Read the model definition and answer for the solid it produces. Units are mm, in the model's axes. A direction names the side the tool comes from. Give positions to 0.01 mm unless a question says otherwise; leave off trailing zeros. Write each loop counter-clockwise with the first axis right and the second up, starting at its lowest first coordinate (ties: lowest second). Pieces come first, ordered by that corner, then holes. Notation, with made-up numbers: M 15,70 L 58,70 A18 cw 58,89 Z; hole C 10,-34.5 d5. An arc over 180 degrees is marked long. Put each result on its own line as item: value.
from build123d import *

# Parameters (mm, degrees)
SKETCH1_R           = 16.66875
BOSS_EXTRUDE1_DEPTH = 3.175
SKETCH2_R           = 16.66875
SKETCH2_R_2         = 13.49375
BOSS_EXTRUDE2_DEPTH = 53.975
SKETCH7_R           = 6.985
CUT_EXTRUDE1_DEPTH  = 62.82084562
SKETCH12_R          = 14.2875
BOSS_EXTRUDE7_DEPTH = 25.4
CUT_EXTRUDE2_REACH  = 63.821
SKETCH9_W           = 12.7
SKETCH9_H           = 11.43
SKETCH9_W_2         = 6.35
SKETCH9_H_2         = 1.6002
SKETCH9_W_3         = 152.4
SKETCH9_H_3         = 3.175
CIRPATTERN2_COUNT   = 4
SKETCH5_R           = 2.5527
SKETCH6_R           = 5.715
CIRPATTERN1_COUNT   = 4


with BuildPart() as part:
    # Sketch1 → Boss-Extrude1 (new body)
    with BuildSketch(Plane(origin=(0, 0, 0), x_dir=(1, 0, 0), z_dir=(0, 1, 0))):
        with Locations(Location((0, 0, 0), (0, 0, 270))):
            Circle(SKETCH1_R)
    extrude(amount=BOSS_EXTRUDE1_DEPTH)

    # Sketch2 → Boss-Extrude2 (add)
    with BuildSketch(Plane(origin=(0, 3.175, 0), x_dir=(1, 0, 0), z_dir=(0, 1, 0))):
        with Locations(Location((0, 0, 0), (0, 0, 270))):
            Circle(SKETCH2_R)
        with Locations(Location((0, 0, 0), (0, 0, 270))):
            Circle(SKETCH2_R_2, mode=Mode.SUBTRACT)
    extrude(amount=BOSS_EXTRUDE2_DEPTH)

    # Sketch7 → Cut-Extrude1 (cut, through all)
    with BuildSketch(Plane.XZ):
        with Locations(Location((0, 0, 0), (0, 0, 270))):
            Circle(SKETCH7_R)
    extrude(amount=-CUT_EXTRUDE1_DEPTH, mode=Mode.SUBTRACT)

    # Sketch12 → Boss-Extrude7 (add)
    with BuildSketch(Plane(origin=(0, 31.75, 0), x_dir=(1, 0, 0), z_dir=(0, 1, 0))):
        Circle(SKETCH12_R)
    extrude(amount=BOSS_EXTRUDE7_DEPTH)

    # Cut-Loft2: read off the stored shape, not the designer's step
    # Cut-Loft2: loft between two sections, ruled curve by curve
    cut_loft2_from = [
        Edge.make_bspline([(-0.505569823, 57.15, -10.307628823), (20.109687823, 57.15, -11.318768468), (21.120827469, 57.15, 9.296489178), (0.505569823, 57.15, 10.307628823), (-20.109687823, 57.15, 11.318768468), (-21.120827469, 57.15, -9.296489178), (-0.505569823, 57.15, -10.307628823)], [0, 0, 0, 0, 0.5, 0.5, 0.5, 1, 1, 1, 1], 3, [1, 0.333333333, 0.333333333, 1, 0.333333333, 0.333333333, 1]),
    ]
    cut_loft2_to = [
        Edge.make_bspline([(-3.365363271, 31.75, -5.384870477), (7.404377683, 31.75, -12.115597019), (14.135104225, 31.75, -1.345856065), (3.365363271, 31.75, 5.384870477), (-7.404377683, 31.75, 12.115597019), (-14.135104225, 31.75, 1.345856065), (-3.365363271, 31.75, -5.384870477)], [0, 0, 0, 0, 0.5, 0.5, 0.5, 1, 1, 1, 1], 3, [1, 0.333333333, 0.333333333, 1, 0.333333333, 0.333333333, 1]),
    ]
    cut_loft2 = Solid(Shell([*[Face.make_surface_from_curves(cut_loft2_from[k], cut_loft2_to[k]) for k in range(1)], Face(Wire(cut_loft2_from)), Face(Wire(cut_loft2_to))]))
    add(cut_loft2, mode=Mode.SUBTRACT)

    # Sketch9 → Cut-Extrude2 (cut, up to next)
    with BuildSketch(Plane(origin=(0, 0, 0), x_dir=(0, -1, 0), z_dir=(-0.7071067811865488, 0, 0.7071067811865464)), mode=Mode.PRIVATE) as cut_extrude2_sk1:
        with Locations((-9.52754, 0)):
            Rectangle(SKETCH9_W, SKETCH9_H)
    cut_extrude2_tool1 = extrude(cut_extrude2_sk1.sketch, amount=-CUT_EXTRUDE2_REACH, mode=Mode.PRIVATE) & part.part
    # Sketch9 → Cut-Extrude2 (cut, up to next)
    with BuildSketch(Plane(origin=(0, 0, 0), x_dir=(0, -1, 0), z_dir=(-0.7071067811865488, 0, 0.7071067811865464)), mode=Mode.PRIVATE) as cut_extrude2_sk2:
        with Locations((-22.225, 0)):
            Rectangle(SKETCH9_W_2, SKETCH9_H_2)
    cut_extrude2_tool2 = extrude(cut_extrude2_sk2.sketch, amount=-CUT_EXTRUDE2_REACH, mode=Mode.PRIVATE) & part.part
    # Sketch9 → Cut-Extrude2 (cut, up to next)
    with BuildSketch(Plane(origin=(0, 0, 0), x_dir=(0, -1, 0), z_dir=(-0.7071067811865488, 0, 0.7071067811865464)), mode=Mode.PRIVATE) as cut_extrude2_sk3:
        with Locations((-101.6, 0)):
            Rectangle(SKETCH9_W_3, SKETCH9_H_3)
    cut_extrude2_tool3 = extrude(cut_extrude2_sk3.sketch, amount=-CUT_EXTRUDE2_REACH, mode=Mode.PRIVATE) & part.part
    cut_extrude2_1 = cut_extrude2_tool1.solids().sort_by_distance((0, 9.52754, 0))[0]
    add(cut_extrude2_1, mode=Mode.SUBTRACT)
    cut_extrude2_2 = cut_extrude2_tool2.solids().sort_by_distance((0, 22.225, 0))[0]
    add(cut_extrude2_2, mode=Mode.SUBTRACT)
    cut_extrude2_3 = cut_extrude2_tool3.solids().sort_by_distance((0, 101.6, 0))[0]
    add(cut_extrude2_3, mode=Mode.SUBTRACT)
    cut_extrude2 = cut_extrude2_1 + cut_extrude2_2 + cut_extrude2_3  # Cut-Extrude2 as one shape, for the pattern or mirror that repeats it

    # CirPattern2: Cut-Extrude2 ×4 about axis
    cirpattern2_axis = Axis((0, 0, 0), (0, 1, 0))
    for i in range(1, CIRPATTERN2_COUNT):
        add(cut_extrude2.rotate(cirpattern2_axis, i * 360 / CIRPATTERN2_COUNT), mode=Mode.SUBTRACT)

    # Sketch5 → Cut-Loft1 section 0
    with BuildSketch(Plane.XZ):
        with Locations((8.255, -8.255)):
            Circle(SKETCH5_R)
    # Sketch6 → Cut-Loft1 section 1
    with BuildSketch(Plane(origin=(0, 3.175, 0), x_dir=(1, 0, 0), z_dir=(0, 1, 0))):
        with Locations((8.255, 8.255)):
            Circle(SKETCH6_R)
    cut_loft1 = loft(mode=Mode.SUBTRACT)

    # CirPattern1: Cut-Loft1 ×4 about axis
    cirpattern1_axis = Axis((0, 0, 0), (0, 1, 0))
    for i in range(1, CIRPATTERN1_COUNT):
        add(cut_loft1.rotate(cirpattern1_axis, i * 360 / CIRPATTERN1_COUNT), mode=Mode.SUBTRACT)


solid = part.part
(1) For a pull along X with two mould halves and no side action, classify faces 5 (the face through (5.8, 9.62, 13.88)), 6 (the face through (-7.2, 0, -0.2)), 7 (the face through (13.88, 9.62, -5.8)) as +X half, -X half, draft (parallel to the pull), parting line (faces both ways), or undercut.
Result:
face 5: +X half
face 6: draft
face 7: undercut
(2) Given pin 1 Ø2 at (y, z) = (34.5, -3) entering from -X; pin 2 Ø12 at (x, y) = (-11.5, 45) entering from +Z; pin 3 Ø8 at (y, z) = (15, 4.5) entering from +X, each flat-ended and moving along its own axis, determine where each tip first touches the part or whether it passes through.
Result:
pin 1: stops at x = -16.55
pin 2: stops at z = 15.74
pin 3: stops at x = 16.66
(3) Which of the six approach directions +Z, -Z, +X, -X, +Y, -Y give full straight-line access (tool end or side, diameter ignored) to faces 1 (the face through (13, 57.15, 0)), 2 (the face through (-10, 31.75, 0)), 3 (the face through (-13.88, 9.62, -5.8)), 4 (the face through (-7.687, 41.497, -9.932))?
Result:
face 1: +Z, -Z, +X, -X, +Y
face 2: none
face 3: -Z
face 4: +Y
(4) Section A-A on y = 4 is taken. Determine the outline of the cut face in (x, z), and give its area (3 significant figures).
Result:
outline: M -15.11,-7.03 L -12.68,-4.6 A13.49 cw -12.68,4.6 L -15.11,7.03 A16.67 ccw Z; M -7.03,-15.11 A16.67 ccw 7.03,-15.11 L 4.6,-12.68 A13.49 cw -4.6,-12.68 Z; M -7.03,15.11 L -4.6,12.68 A13.49 cw 4.6,12.68 L 7.03,15.11 A16.67 ccw Z; M 12.68,-4.6 L 15.11,-7.03 A16.67 ccw 15.11,7.03 L 12.68,4.6 A13.49 cw Z
area: 152 mm²
(5) Section B-B on y = 52.5 is taken. Give the number of separate pieces and of enclosed holes in the cut face, and give its area (3 significant figures).
Result:
separate pieces: 4
enclosed holes: 0
area: 500 mm²
(6) Straight lines are drawn through the part: line 1 along Z through (x, y) = (0, 23); line 2 along Z through (x, y) = (-9, 54.5). For each, find the intervals that lie inside material, in ascending order. Write a range as from..to.
Result:
line 1: z = -16.67..-13.49, 13.49..16.67
line 2: z = -14.03..-11.25, -6.75..-3.95, 3.95..6.75, 11.25..14.03
